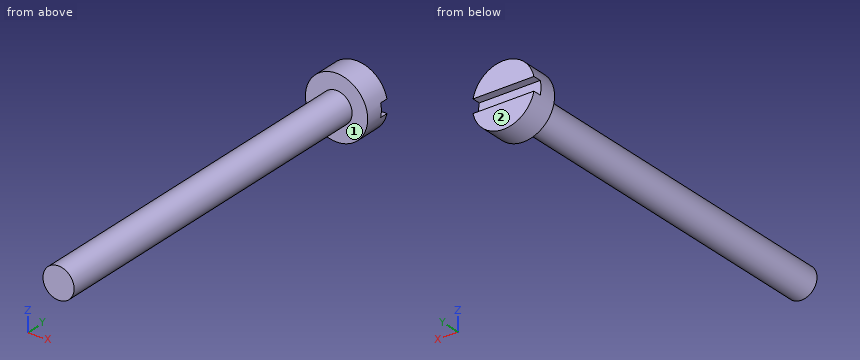
Solid Edge part; units mm, degrees
sketch "Sketch1" plane through (0, 0, 0) normal (0, -1, 0) x (1, 0, 0)
  circle A0 centre (0, 0) radius 1.5
extrude "Protrusion1" add sketch "Sketch1" against normal blind 35
sketch "Sketch2" plane through (0, 35, 0) normal (0, 1, 0) x (1, 0, 0)
  circle A0 centre (0, 0) radius 3
extrude "ExtrudedProtrusion_2" add sketch "Sketch2" along normal blind 2.52
sketch "Sketch3" plane through (0, 37.52, 0) normal (0, 1, 0) x (-1, 0, 0)
  line L0 (-2.9311, 0.6393) -> (2.9311, 0.6393)
  arc A0 (2.9311, 0.6393) -> (2.9311, -0.6393) centre (0, 0) cw
  line L1 (2.9311, -0.6393) -> (-2.9311, -0.6393)
  arc A1 (-2.9311, -0.6393) -> (-2.9311, 0.6393) centre (0, 0) cw
extrude "ExtrudedCutout_1" cut sketch "Sketch3" against normal blind 0.8
cosmetic_thread "Thread1"
properties material "Nylon, general purpose"
Design review of the part built by this model. Coordinates are the model's own, in mm. Face numbers are marked on the shaded views. A direction names the side the tool comes from. Coordinates: 2 decimals unless noted, no trailing zeros. Write each loop counter-clockwise with the first axis right and the second up, starting at its lowest first coordinate (ties: lowest second). Pieces come first, ordered by that corner, then holes.
1) Add section C-C (y = 14). Write out the cut boundary in (x, z), plus the area to 3 significant figures.
2) Add section A-A (x = 0). Write out the cut boundary in (y, z), plus the area to 3 significant figures.
3) Machinability: for the marked faces 1 and 2, which of the approach directions +Z, -Z, +X, -X, +Y, -Y give a long, thin tool a straight path to every point of the face, cutting with its end or side? Answer none if there is none.
4) Insertion check: pin 1 (1.5 mm diameter, centred on x = 0, z = 0.5, fed in from +Y); pin 2 (2 mm diameter, centred on x = 1.5, y = 7, fed in from +Z); pin 3 (1.5 mm diameter, centred on y = 11, z = -2, fed in from -X); pin 4 (1 mm diameter, centred on x = -0.5, y = 13.5, fed in from +Z). Each pin has a flat end and moves straight along its axis. Give the tip position at first contact, or say it passes through.
5) To check wall thickness, follow L1, parallel to Y at x = -0.1, z = 2; L2, parallel to X at y = 8, z = -0.1; L3, parallel to Y at x = -1.7, z = 0.15. State the ranges of each line that lie inside material, in increasing order.
6) Add section B-B (z = 0.95). Write out the cut boundary in (x, y).
7) Add section D-D (x = -2.1). Write out the cut boundary in (y, z), plus the area to 3 significant figures.
Check result:
1. outline: circle Ø3 at (0, 0)
1. area: 7.07 mm2
2. outline: (0, -1.5) - (35, -1.5) - (35, -3) - (37.52, -3) - (37.52, -0.64) - (36.72, -0.64) - (36.72, 0.64) - (37.52, 0.64) - (37.52, 3) - (35, 3) - (35, 1.5) - (0, 1.5) - close
2. area: 119 mm2
3. face 1: -Y
3. face 2: +Z, -Z, +X, -X, +Y
4. pin 1: stops at y = 37.52
4. pin 2: stops at z = 1.41
4. pin 3: stops at x = -0.83
4. pin 4: stops at z = 1.5
5. L1: y = 35 to 37.52
5. L2: x = -1.5 to 1.5
5. L3: y = 35 to 36.72
6. outline: (-2.85, 35) - (-1.16, 35) - (-1.16, 0) - (1.16, 0) - (1.16, 35) - (2.85, 35) - (2.85, 37.52) - (-2.85, 37.52) - close
7. outline: (35, -2.14) - (37.52, -2.14) - (37.52, -0.64) - (36.72, -0.64) - (36.72, 0.64) - (37.52, 0.64) - (37.52, 2.14) - (35, 2.14) - close
7. area: 9.77 mm2
